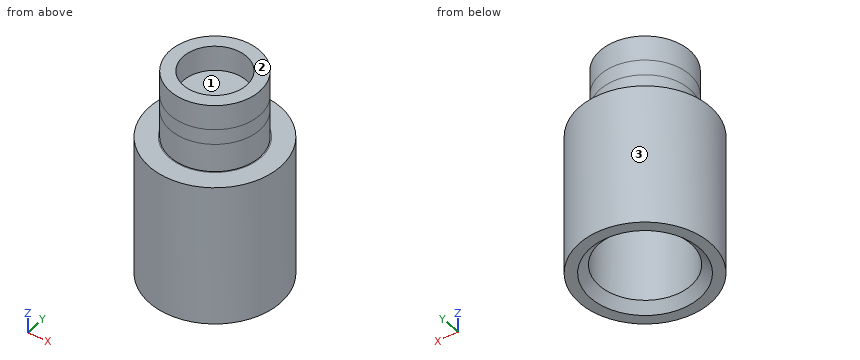
```python
from build123d import *

# Parameters (mm, degrees)
F0_R        = 6
F0_R_2      = 4.2
F1_DEPTH    = 13
F2_R        = 4.1
F2_R_2      = 2.9
F3_DEPTH    = 6.3
F4_R        = 4.2
F4_R_2      = 2.9
F5_DEPTH    = 3
F6_S5_R     = 4.2
F6_T6_DEPTH = 9
F7_SIZE     = 0.8
F9_R        = 4.1
F10_DEPTH   = 0.7


# Not quite as in the source:
# - a fillet or chamfer that OpenCascade refuses, or shapes differently, is made with other operations: its cross-section is extruded or revolved along the edge and cut away or added


with BuildPart() as f1:
    # F0 (on Top) → F1 (new body)
    with BuildSketch(Plane.XY):
        Circle(F0_R)
        Circle(F0_R_2, mode=Mode.SUBTRACT)
    extrude(amount=F1_DEPTH)



with BuildPart() as f3:
    # F2 (on face) → F3 (new body)
    with BuildSketch(Plane.XY.offset(13)):
        Circle(F2_R)
        Circle(F2_R_2, mode=Mode.SUBTRACT)
    extrude(amount=F3_DEPTH)


with BuildPart() as f1_1:
    add(f1.part)

    add(f3.part)  # F5 merges F3
    # F4 (on face) → F5 (join)
    with BuildSketch(Plane.XY.offset(13)):
        Circle(F4_R)
        Circle(F4_R_2, mode=Mode.SUBTRACT)
    extrude(amount=-F5_DEPTH)

    # F6: chamfer of 2 on 1 edges, made by hand


with BuildPart() as f6_tool2:
    # F6_s3 → F6_t4 (revolve)
    with BuildSketch(Plane.XZ):
        Polygon((2.9, 12), (4.9, 10), (2.9, 10), align=None)
    revolve(axis=Axis((0, 0, 10), (0, 0, 1)))

    # F6_s5 → F6_t6 (intersect, symmetric)
    with BuildSketch(Plane.XY.offset(11)):
        Circle(F6_S5_R)
    extrude(amount=F6_T6_DEPTH, both=True, mode=Mode.INTERSECT)


with BuildPart() as f1_2:
    add(f1_1.part)

    # F6_t1: cut F6_tool2
    add(f6_tool2.part, mode=Mode.SUBTRACT)

    # F7
    f7_edges = [f1_2.edges().sort_by_distance(p)[0] for p in [
        (-4.2, 0, 0),
    ]]
    chamfer(f7_edges, length=F7_SIZE)

    # F9 (on offset) → F10 (join, symmetric)
    with BuildSketch(Plane.XY.offset(16.3)):
        Circle(F9_R)
    extrude(amount=F10_DEPTH, both=True)


solid = f1_2.part
```
The listing builds one solid part. Answer for the finished solid, in the listing's coordinates (mm). Face numbers are marked on the shaded views. Round coordinates to 2 decimals unless told otherwise and drop trailing zeros. Loops run counter-clockwise (first coordinate to the right, second up) from the corner with the lowest first, then second, coordinate; pieces in that order, holes last.
1) Given P1, Ø2, axis at y = -3, z = 13, coming from the +X side; P2, Ø4.5, axis at x = 1.5, y = 0.5, coming from the -Z side; P3, Ø1.5, axis at x = 3, z = 8.5, coming from the -Y side; P4, Ø4.5, axis at x = 1, y = -1.5, coming from the +Z side, each flat-ended and moving along its own axis, determine where each tip first touches the part or whether it passes through.
Outcome:
P1: stops at x = 5.66
P2: stops at z = 11.07
P3: stops at y = -5.56
P4: stops at z = 19.3
2) For a pull along X with two mould halves and no side action, classify the marked faces 1, 2 and 3 as released by +X, released by -X, zero draft, split by the parting line, or undercut.
Outcome:
face 1: undercut
face 2: zero draft
face 3: split by the parting line
3) A cutting plane is placed at C-C on z = 13.75. Determine the outline of the cut face in (x, y), plus the area to 3 significant figures.
Outcome:
outline: circle Ø8.2 at (0, 0); hole circle Ø5.8 at (0, 0)
area: 26.4 mm2
4) A cutting plane is placed at D-D on z = 6.75. Determine the outline of the cut face in (x, y), plus the area to 3 significant figures.
Outcome:
outline: circle Ø12 at (0, 0); hole circle Ø8.4 at (0, 0)
area: 57.7 mm2
5) A cutting plane is placed at A-A on y = 0. Determine the outline of the cut face in (x, z), plus the area to 3 significant figures.
Outcome:
outline: (-6, 0) - (-5, 0) - (-4.2, 0.8) - (-4.2, 10.7) - (-2.9, 12) - (-2.9, 15.6) - (2.9, 15.6) - (2.9, 12) - (4.2, 10.7) - (4.2, 0.8) - (5, 0) - (6, 0) - (6, 13) - (4.1, 13) - (4.1, 19.3) - (2.9, 19.3) - (2.9, 17) - (-2.9, 17) - (-2.9, 19.3) - (-4.1, 19.3) - (-4.1, 13) - (-6, 13) - close
area: 73.7 mm2
6) Consider line 1 (Y direction, x = 0, z = 18.3); line 2 (Z direction, x = 2, y = 0); line 3 (Z direction, x = 3, y = -5). Determine where each line is inside the solid, lowest interval first.
Outcome:
line 1: y = -4.1 to -2.9, 2.9 to 4.1
line 2: z = 15.6 to 17
line 3: z = 0 to 13
